Here's how the part is built. I have some questions about the finished solid (model axes, mm). Round coordinates to 2 decimals unless told otherwise and drop trailing zeros. Answer as CSV lines item,"result".
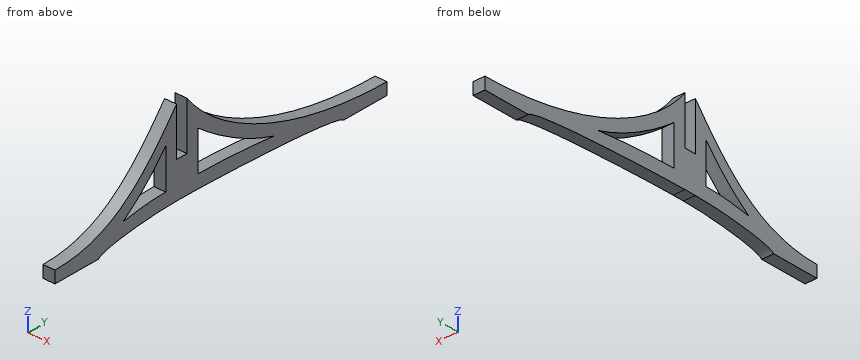
from build123d import *

# Parameters (mm, degrees)
F0_W     = 2.4
F0_H     = 15
F1_DEPTH = 5


# Not quite as in the source:
# - a feature names something its author has since deleted; it is built from what else it names


with BuildPart() as f1:
    # F0 (on Right) → F1 (new body)
    with BuildSketch(Plane.YZ):
        with Locations((-1.2, 12.5)):
            Rectangle(F0_W, F0_H)
        with Locations((1.2, 12.5)):
            Rectangle(F0_W, F0_H)
        with BuildLine():
            Line((2.4, 20), (2.4, 5))
            add(Edge.make_bspline(
                [(74.7971267972, 0), (71.3879865607, 3.4156564958), (16.494217181, 5), (2.4, 5)],
                knots=[0, 0, 0, 0, 72.5695801868, 72.5695801868, 72.5695801868, 72.5695801868], degree=3))
            Line((74.7971267972, 0), (94.7971267972, 0))
            Line((94.7971267972, 0), (94.7971267972, 5))
            add(Edge.make_bspline(
                [(2.4, 40), (16.6215170175, 20.5895993859), (51.1409416795, 5), (94.7971267972, 5)],
                knots=[0, 0, 0, 0, 98.8039930387, 98.8039930387, 98.8039930387, 98.8039930387], degree=3))
            Line((2.4, 40), (2.4, 20))
        make_face()
        with BuildLine():
            add(Edge.make_bspline(
                [(7.4, 27.0048175007), (7.4282917172, 21.6293986887), (7.3717082828, 15.8260287717), (7.4, 10.4506099597)],
                knots=[0, 0, 0, 0, 16.554207541, 16.554207541, 16.554207541, 16.554207541], degree=3))
            add(Edge.make_bspline(
                [(42.5923541188, 8.5242791101), (28.9157964289, 12.3093035072), (16.1028206348, 20.2473960817), (7.4, 27.0048175007)],
                knots=[0, 0, 0, 0, 39.7496174526, 39.7496174526, 39.7496174526, 39.7496174526], degree=3))
            add(Edge.make_bspline(
                [(7.4, 10.4506099597), (17.3497335032, 10.4361297563), (31.9942831993, 9.6850190312), (42.5923541188, 8.5242791101)],
                knots=[0, 0, 0, 0, 35.2450356641, 35.2450356641, 35.2450356641, 35.2450356641], degree=3))
        make_face(mode=Mode.SUBTRACT)
        with BuildLine():
            add(Edge.make_bspline(
                [(-2.4, 5), (-13.9117193222, 5), (-35.8368966605, 2.8542873915), (-38.5822232689, 0)],
                knots=[0, 0, 0, 0, 36.5260630329, 36.5260630329, 36.5260630329, 36.5260630329], degree=3))
            Line((-2.4, 5), (-2.4, 20))
            Line((-2.4, 20), (-2.4, 30.4898899049))
            Line((-2.4, 30.4898899049), (-2.4, 40))
            add(Edge.make_bspline(
                [(-58.5822232689, 5), (-32.4707888067, 5), (-18.0997792631, 19.8830608279), (-2.4, 40)],
                knots=[0, 0, 0, 0, 66.1924634036, 66.1924634036, 66.1924634036, 66.1924634036], degree=3))
            Line((-58.5822232689, 5), (-58.5822232689, 0))
            Line((-58.5822232689, 0), (-38.5822232689, 0))
        make_face()
        with BuildLine():
            add(Edge.make_bspline(
                [(-7.4, 27.0048175007), (-14.9471499026, 18.3299258351), (-18.6816509813, 14.8076107726), (-27.100559324, 8.5242791101)],
                knots=[0, 0, 0, 0, 27.0118925084, 27.0118925084, 27.0118925084, 27.0118925084], degree=3))
            add(Edge.make_bspline(
                [(-7.4, 27.0048175007), (-7.4600156685, 21.4867483204), (-7.3399843315, 15.96867914), (-7.4, 10.4506099597)],
                knots=[0, 0, 0, 0, 16.554207541, 16.554207541, 16.554207541, 16.554207541], degree=3))
            add(Edge.make_bspline(
                [(-27.100559324, 8.5242791101), (-19.2162878811, 9.7881155089), (-14.8515102789, 10.4084629565), (-7.4, 10.4506099597)],
                knots=[0, 0, 0, 0, 19.7945140941, 19.7945140941, 19.7945140941, 19.7945140941], degree=3))
        make_face(mode=Mode.SUBTRACT)
    extrude(amount=F1_DEPTH)


solid = f1.part
Item 1: Will these pins go through, and if not, where does the flat tip stop? pin 1 (2.5 mm diameter, centred on x = 2, y = 0.5, fed in from +Z); pin 2 (1.5 mm diameter, centred on x = 1.5, y = 28, fed in from +Z); pin 3 (1.5 mm diameter, centred on x = 3.5, z = 35, fed in from +Y); pin 4 (8 mm diameter, centred on y = 17.5, z = 27.5, fed in from -X).
Results found:
pin 1,"stops at z = 20"
pin 2,"stops at z = 19.93"
pin 3,"stops at y = 7.32"
pin 4,"stops at x = 0"
Item 2: Suppose I cut it at A-A, the plane x = 0.85. State how many separate pieces and enclosed holes the cut face has, then the cut area to 3 significant figures.
Results found:
separate pieces,"1"
enclosed holes,"2"
area,"1,560 mm²"
Item 3: I need wall thicknesses on L1, parallel to Y at x = 3.15, z = 17; L2, parallel to Y at x = 4.4, z = 18.5; L3, parallel to Y at x = 3, z = 26.5 (3 decimals). Which ranges of each line are inside material? Lowest first, please.
Results found:
L1,"y = -23.85 to -16.78, -7.39 to 7.4, 22.5 to 33.34"
L2,"y = -22.01 to -15.23, -7.4 to 7.4, 19.9 to 30.1"
L3,"y = -13.705 to -7.84, -7.405 to -2.4, 2.4 to 7.402, 8.055 to 16.476"
